from build123d import *

# Parameters (mm, degrees)
F0_W     = 87
F0_H     = 170
F1_DEPTH = 5
F2_W     = 15
F2_H     = 30
F3_DEPTH = 25


with BuildPart() as f1:
    # F0 (on Front) → F1 (new body)
    with BuildSketch(Plane.XZ):
        with Locations((43.5, 85)):
            Rectangle(F0_W, F0_H)
    extrude(amount=F1_DEPTH)

    # F2 (on face) → F3 (cut)
    with BuildSketch(Plane.XZ.offset(5)):
        with BuildLine():
            ThreePointArc((10, 7), (8.93934, 6.56066), (8.5, 5.5))
            Line((8.5, 5.5), (10, 5.5))
            Line((10, 5.5), (10, 7))
        make_face()
        with BuildLine():
            ThreePointArc((11.5, 51.5), (8.93934, 52.56066), (10, 50))
            ThreePointArc((10, 50), (11.06066, 50.43934), (11.5, 51.5))
        make_face()
        with BuildLine():
            Line((10, 5.5), (8.5, 5.5))
            ThreePointArc((8.5, 5.5), (10, 4), (11.5, 5.5))
            ThreePointArc((11.5, 5.5), (11.06066, 6.56066), (10, 7))
            Line((10, 7), (10, 5.5))
        make_face()
        with BuildLine():
            ThreePointArc((77, 7), (75.93934, 4.43934), (78.5, 5.5))
            Line((78.5, 5.5), (77, 5.5))
            Line((77, 5.5), (77, 7))
        make_face()
        with BuildLine():
            Line((77, 5.5), (78.5, 5.5))
            ThreePointArc((78.5, 5.5), (78.06066, 6.56066), (77, 7))
            Line((77, 7), (77, 5.5))
        make_face()
        with BuildLine():
            ThreePointArc((78.5, 51.5), (75.93934, 52.56066), (77, 50))
            ThreePointArc((77, 50), (78.06066, 50.43934), (78.5, 51.5))
        make_face()
        with BuildLine():
            ThreePointArc((11.5, 164.5), (10, 166), (8.5, 164.5))
            Line((8.5, 164.5), (10, 164.5))
            Line((10, 164.5), (10, 163))
            ThreePointArc((10, 163), (11.06066, 163.43934), (11.5, 164.5))
        make_face()
        with BuildLine():
            ThreePointArc((11.5, 118.5), (11.06066, 119.56066), (10, 120))
            ThreePointArc((10, 120), (8.93934, 117.43934), (11.5, 118.5))
        make_face()
        with BuildLine():
            Line((10, 164.5), (8.5, 164.5))
            ThreePointArc((8.5, 164.5), (8.93934, 163.43934), (10, 163))
            Line((10, 163), (10, 164.5))
        make_face()
        with BuildLine():
            ThreePointArc((77, 163), (78.06066, 163.43934), (78.5, 164.5))
            Line((78.5, 164.5), (77, 164.5))
            Line((77, 164.5), (77, 163))
        make_face()
        with BuildLine():
            Line((77, 164.5), (78.5, 164.5))
            ThreePointArc((78.5, 164.5), (75.93934, 165.56066), (77, 163))
            Line((77, 163), (77, 164.5))
        make_face()
        with BuildLine():
            ThreePointArc((78.5, 118.5), (78.06066, 119.56066), (77, 120))
            ThreePointArc((77, 120), (75.93934, 117.43934), (78.5, 118.5))
        make_face()
        with Locations((66, 85)):
            Rectangle(F2_W, F2_H)
        with Locations((21, 85)):
            Rectangle(F2_W, F2_H)
        with BuildLine():
            ThreePointArc((32.5, 121), (32.06066, 122.06066), (31, 122.5))
            ThreePointArc((31, 122.5), (29.93934, 119.93934), (32.5, 121))
        make_face()
        with BuildLine():
            ThreePointArc((32.5, 129), (29.93934, 130.06066), (31, 127.5))
            ThreePointArc((31, 127.5), (32.06066, 127.93934), (32.5, 129))
        make_face()
        with BuildLine():
            ThreePointArc((57.5, 129), (54.93934, 130.06066), (56, 127.5))
            ThreePointArc((56, 127.5), (57.06066, 127.93934), (57.5, 129))
        make_face()
        with BuildLine():
            ThreePointArc((57.5, 121), (57.06066, 122.06066), (56, 122.5))
            ThreePointArc((56, 122.5), (54.93934, 119.93934), (57.5, 121))
        make_face()
        with BuildLine():
            ThreePointArc((57.5, 49), (54.93934, 50.06066), (56, 47.5))
            ThreePointArc((56, 47.5), (57.06066, 47.93934), (57.5, 49))
        make_face()
        with BuildLine():
            ThreePointArc((57.5, 41), (57.06066, 42.06066), (56, 42.5))
            ThreePointArc((56, 42.5), (54.93934, 39.93934), (57.5, 41))
        make_face()
        with BuildLine():
            ThreePointArc((32.5, 41), (32.06066, 42.06066), (31, 42.5))
            ThreePointArc((31, 42.5), (29.93934, 39.93934), (32.5, 41))
        make_face()
        with BuildLine():
            ThreePointArc((32.5, 49), (29.93934, 50.06066), (31, 47.5))
            ThreePointArc((31, 47.5), (32.06066, 47.93934), (32.5, 49))
        make_face()
    extrude(amount=-F3_DEPTH, mode=Mode.SUBTRACT)


solid = f1.part
Geometry: final body of the model. Coordinates: model frame, mm. A direction names the side the tool comes from. Give positions to 0.01 mm unless a question says otherwise; leave off trailing zeros. Order: outer loops, then holes, each group sorted by start corner. A loop starts at its lowest first (then second) coordinate and runs counter-clockwise, first axis right, second up. Notation, with made-up numbers: (-2.75, -9) -> (48.25, -9) arc R18 ccw to (48.25, 4) -> close; hole circle Ø1 at (4, 61.25). An arc over 180 degrees is marked (long way). Put each result on its own line as item: value.
Q1. Material intervals for L1, parallel to Z at x = 10, y = -2.75; L2, parallel to X at y = -1.75, z = 51.5; L3, parallel to Z at x = 56, y = -2.2, sorted ascending.
Here are the results:
L1: z = 0 to 4, 7 to 50, 53 to 117, 120 to 163, 166 to 170
L2: x = 0 to 8.5, 11.5 to 75.5, 78.5 to 87
L3: z = 0 to 39.5, 42.5 to 47.5, 50.5 to 119.5, 122.5 to 127.5, 130.5 to 170
Q2. Reachability of faces 4 (the face through (66, -3, 70)), 5 (the face through (43, -5, 86)) from +Z, -Z, +X, -X, +Y, -Y: full face, straight path, thin tool, end or side. Return the list, or none.
Here are the results:
face 4: +Y, -Y
face 5: +Z, -Z, +X, -X, -Y
Q3. Draft query along Z for faces 1 (the face through (87, -2, 84)), 2 (the face through (43, -2, 0)), 3 (the face through (13.5, -3, 85)). Return one class per face: released by +Z, released by -Z, zero draft, split by the parting line, or undercut.
Here are the results:
face 1: zero draft
face 2: released by -Z
face 3: undercut
Q4. Section A-A, the plane x = 20. Return loops of the section in (y, z), then the cut area to 3 significant figures.
Here are the results:
outline: (-5, 0) -> (0, 0) -> (0, 70) -> (-5, 70) -> close; (-5, 100) -> (0, 100) -> (0, 170) -> (-5, 170) -> close
area: 700 mm^2
Q5. Section B-B, the plane y = -3.85. Count the separate pieces of the cut face and the enclosed holes in it, then the cut area to 3 significant figures.
Here are the results:
separate pieces: 1
enclosed holes: 18
area: 13,800 mm^2
Q6. Pin query (flat end, axial travel): pin 1 (4 mm diameter, centred on x = 56, z = 121, fed in from -Y). Return the tip coordinate at first contact, or that it passes through.
Here are the results:
pin 1: stops at y = -5
